Here's how the part is built. I have some questions about the finished solid (model axes, mm). Round coordinates to 2 decimals unless told otherwise and drop trailing zeros. Order: outer loops, then holes, each group sorted by start corner. A loop starts at its lowest first (then second) coordinate and runs counter-clockwise, first axis right, second up. Notation, with made-up numbers: (-12.5, -30) -> (36.5, -30) arc R12 cw to (36.5, -16) -> close; hole circle Ø8 at (43, 36). An arc over 180 degrees is marked (long way). Answer in a Markdown table with one row per item.
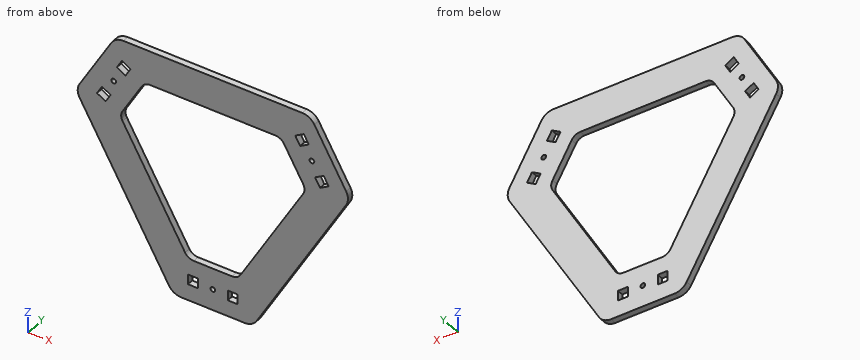
```python
from build123d import *

# Parameters (mm, degrees)
BOSS_EXTRUDE1_DEPTH = 4.0386
SKETCH2_R           = 1.5
SKETCH2_W           = 6.35
SKETCH2_H           = 6.35
CUT_EXTRUDE1_DEPTH  = 5.0386
CIRPATTERN1_COUNT   = 3
FILLET1_R           = 8.89
FILLET2_R           = 6.35


with BuildPart() as part:
    # Sketch1 → Boss-Extrude1 (new body)
    with BuildSketch(Plane(origin=(0, 0, 0), x_dir=(1, 0, 0), z_dir=(0, 1, 0))):
        Polygon((-25.4, 86.518604358), (25.4, 86.518604358), (87.627309274, -21.262256923), (62.227309274, -65.256347435), (-62.227309274, -65.256347435), (-87.627309274, -21.262256923), align=None)
        Polygon((-15.875, 59.51410253), (15.875, 59.51410253), (59.478224675, -16.00889798), (43.603224675, -43.50520455), (-43.603224675, -43.50520455), (-59.478224675, -16.00889798), align=None, mode=Mode.SUBTRACT)
    extrude(amount=BOSS_EXTRUDE1_DEPTH)

    # Sketch2 → Cut-Extrude1 (cut, through all)
    with BuildSketch(Plane(origin=(0, 4.0386, 0), x_dir=(1, 0, 0), z_dir=(0, 1, 0))):
        with Locations((0, 73.025)):
            Circle(SKETCH2_R)
        with Locations((12.7, 73.025)):
            Rectangle(SKETCH2_W, SKETCH2_H)
        with Locations((-12.7, 73.025)):
            Rectangle(SKETCH2_W, SKETCH2_H)
    cut_extrude1 = extrude(amount=-CUT_EXTRUDE1_DEPTH, mode=Mode.SUBTRACT)

    # CirPattern1: Cut-Extrude1 ×3 about axis
    cirpattern1_axis = Axis((0, 0, 0), (0, 1, 0))
    for i in range(1, CIRPATTERN1_COUNT):
        add(cut_extrude1.rotate(cirpattern1_axis, i * 360 / CIRPATTERN1_COUNT), mode=Mode.SUBTRACT)

    # Fillet1
    fillet1_edges = [part.edges().sort_by_distance(p)[0] for p in [
        (-25.4, 2.0193, -86.518604358),
        (25.4, 2.0193, -86.518604358),
        (87.627309274, 2.0193, 21.262256923),
        (62.227309274, 2.0193, 65.256347435),
        (-62.227309274, 2.0193, 65.256347435),
        (-87.627309274, 2.0193, 21.262256923),
    ]]
    fillet(fillet1_edges, radius=FILLET1_R)

    # Fillet2
    fillet2_edges = [part.edges().sort_by_distance(p)[0] for p in [
        (-15.875, 2.0193, -59.51410253),
        (-59.478224675, 2.0193, 16.00889798),
        (-43.603224675, 2.0193, 43.50520455),
        (43.603224675, 2.0193, 43.50520455),
        (59.478224675, 2.0193, 16.00889798),
        (15.875, 2.0193, -59.51410253),
    ]]
    fillet(fillet2_edges, radius=FILLET2_R)


solid = part.part
```
1. Please list where these lines run through material, in increasing order: line 1 along Z through (x, y) = (0, 1.75) (3 decimals); line 2 along Z through (x, y) = (-40, 3.2); line 3 along X through (y, z) = (1.15, 25).
Numbers:
| item | result |
|---|---|
| line 1 | z = -86.519 to -74.525, -71.525 to -59.514, 43.505 to 65.256 |
| line 2 | z = -61.23 to -17.73, 43.5 to 65.26 |
| line 3 | x = -85.43 to -73.55, -66.22 to -54.29, 54.29 to 66.22, 73.55 to 85.43 |
2. Suppose I cut it at A-A on x = -23. Write out the boundary of the cut face in (y, z), then the cut area to 3 significant figures.
Numbers:
| item | result |
|---|---|
| outline | (0, -86.09) -> (4.04, -86.09) -> (4.04, -47.17) -> (0, -47.17) -> close; (0, 43.51) -> (4.04, 43.51) -> (4.04, 65.26) -> (0, 65.26) -> close |
| area | 245 mm2 |
3. Suppose I cut it at B-B on z = -39.5. Write out the boundary of the cut face in (x, y), then the cut area to 3 significant figures.
Numbers:
| item | result |
|---|---|
| outline | (-52.55, 0) -> (-27.43, 0) -> (-27.43, 4.04) -> (-52.55, 4.04) -> close; (27.43, 0) -> (52.55, 0) -> (52.55, 4.04) -> (27.43, 4.04) -> close |
| area | 203 mm2 |
4. For pin 1 Ø8 at (x, z) = (7.5, 36.5) entering from +Y; pin 2 Ø1.2 at (y, z) = (1.5, -72.5) entering from -X; pin 3 Ø2 at (y, z) = (1.5, -72) entering from +X; pin 4 Ø5 at (x, z) = (-63.24, 36.51) entering from +Y, each with a flat end and sliding along its axis, tell me the tip position at first contact or that it passes through.
Numbers:
| item | result |
|---|---|
| pin 1 | passes through |
| pin 2 | stops at x = -33.84 |
| pin 3 | stops at x = 34.36 |
| pin 4 | stops at y = 4.04 |
5. Suppose I cut it at C-C on y = 3.4. State how many separate pieces and enclosed holes the cut face has, then the cut area to 3 significant figures.
Numbers:
| item | result |
|---|---|
| separate pieces | 1 |
| enclosed holes | 10 |
| area | 9,970 mm2 |
